Build history of the part. All positions in model axes, mm. Face numbers are marked on the shaded views. A direction names the side the tool comes from. Round coordinates to 2 decimals unless told otherwise and drop trailing zeros. Order: outer loops, then holes, each group sorted by start corner. A loop starts at its lowest first (then second) coordinate and runs counter-clockwise, first axis right, second up. Notation, with made-up numbers: (43, 41.5) - (93, 41.5) arc R16 cw to (93, 48.5) - close; hole circle Ø11 at (-34, 29). An arc over 180 degrees is marked (long way). Write each question's results on one line, items separated by ' | '. Start each with the question number.
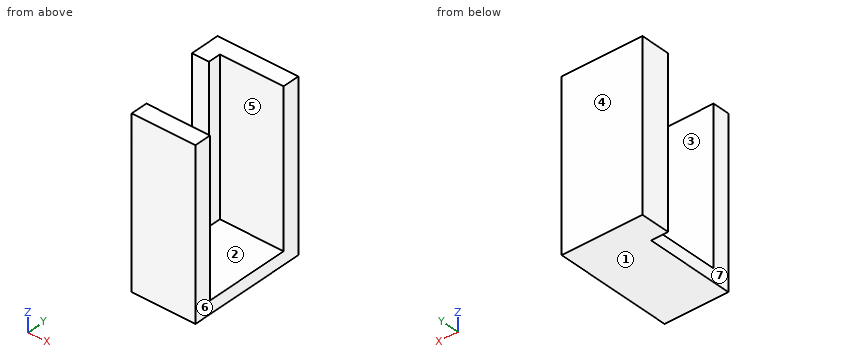
Solid Edge part; units mm, degrees
sketch "Sketch1" plane through (0, 0, 0) normal (0, 0, 1) x (1, 0, 0)
  line L0 (-3.75, -7) -> (3.75, -7)
  line L1 (3.75, -7) -> (3.75, 7)
  line L2 (3.75, 7) -> (-3.75, 7)
  line L3 (-3.75, 7) -> (-3.75, -7)
  dimension "D1" = 3.75
  dimension "D2" = 3.75
extrude "Protrusion1" add sketch "Sketch1" along normal blind 1.5
sketch "Sketch2" plane through (0, 0, 1.5) normal (0, 0, 1) x (1, 0, 0)
  line L0 (-3.75, 7) -> (3.75, 7)
  line L1 (3.75, 7) -> (3.75, 5)
  line L2 (3.75, 5) -> (-3.75, 5)
  line L3 (-3.75, 5) -> (-3.75, 7)
  line L4 (-3.75, -7) -> (3.75, -7)
  line L5 (3.75, -7) -> (3.75, -5)
  line L6 (3.75, -5) -> (-3.75, -5)
  line L7 (-3.75, -5) -> (-3.75, -7)
  dimension "D1" = 3.75
  dimension "D2" = 3.75
extrude "Extrusionsausprägung_2" add sketch "Sketch2" along normal blind 18
sketch "Sketch3" plane through (0, 6, 19.5) normal (0, 0, 1) x (0, 1, 0)
  line L0 (1, 3.75) -> (-2.5, 3.75)
  line L1 (-2.5, 3.75) -> (-2.5, 5.75)
  line L2 (-2.5, 5.75) -> (1, 5.75)
  line L3 (1, 5.75) -> (1, 3.75)
  dimension "D1" = 1
  dimension "D2" = 2.5
extrude "Protrusion2" add sketch "Sketch3" against normal up to vertex (19.5 mm away)
properties material "Nylon, allgemein"
1. Flat gauge pins, fed straight in: pin 1 Ø2 at (x, y) = (0.5, 1.5) entering from +Z; pin 2 Ø1 at (x, z) = (-4.5, 11.5) entering from -Y; pin 3 Ø1.5 at (x, y) = (-2, 2.5) entering from -Z; pin 4 Ø8 at (y, z) = (-5, 11.5) entering from -X. Where does each tip first touch, or does it go through?
2. Cut at D-D (x = -4.75). List the corners of the cut face in (y, z), plus the area to 4 significant figures.
3. Cut at C-C (y = -4). List the corners of the cut face in (x, z).
4. 3-axis set-ups, long thin cutter, end or side, ignore diameter. For the marked faces 5, 6 and 7: which of +Z, -Z, +X, -X, +Y, -Y reach the whole face in a straight line?
5. Cut at B-B (x = 3). List the corners of the cut face in (y, z).
6. Cut at A-A (z = 11). List the corners of the cut face in (x, y).
7. Mould opens along Y. For the marked faces 1, 2, 3 and 4 say: pulls with the +Y half, pulls with the -Y half, needs draft (parallel to the pull), parting line crosses it, or undercut.
8. Wall check: line 1 (Y direction, x = 0, z = 18.5); line 2 (Y direction, x = -4, z = 10.75); line 3 (X direction, y = 1.25, z = 1). Give the ranges that are in metal, low to high. Write a range as from..to.
A:
1) pin 1: stops at z = 1.5 | pin 2: stops at y = 3.5 | pin 3: stops at z = 0 | pin 4: stops at x = -3.75
2) outline: (3.5, 0) - (7, 0) - (7, 19.5) - (3.5, 19.5) - close | area: 68.25 mm^2
3) outline: (-3.75, 0) - (3.75, 0) - (3.75, 1.5) - (-3.75, 1.5) - close
4) face 5: +Z, +X | face 6: +Z, -Z, +X, +Y, -Y | face 7: +Z, -Z, -X, -Y
5) outline: (-7, 0) - (7, 0) - (7, 19.5) - (5, 19.5) - (5, 1.5) - (-5, 1.5) - (-5, 19.5) - (-7, 19.5) - close
6) outline: (-5.75, 3.5) - (-3.75, 3.5) - (-3.75, 5) - (3.75, 5) - (3.75, 7) - (-5.75, 7) - close; (-3.75, -7) - (3.75, -7) - (3.75, -5) - (-3.75, -5) - close
7) face 1: needs draft | face 2: undercut | face 3: undercut | face 4: pulls with the +Y half
8) line 1: y = -7..-5, 5..7 | line 2: y = 3.5..7 | line 3: x = -3.75..3.75
